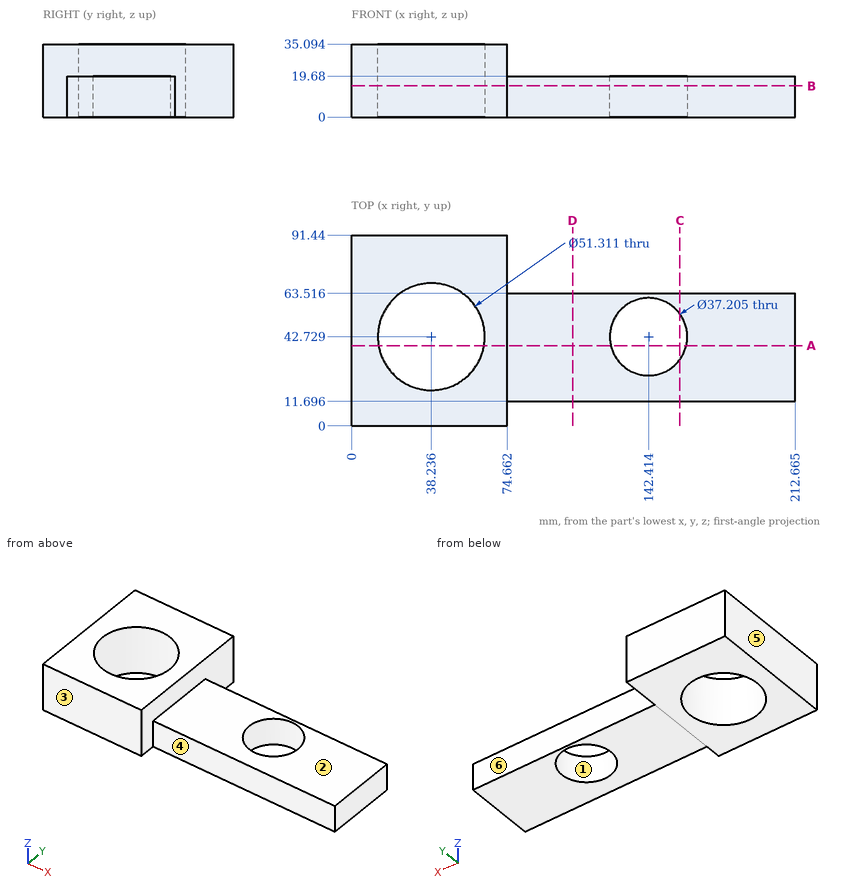
The figure shows three views and two pictorial views of one solid part (mm, origin at its lowest corner). Answer the questions. A direction names the side the tool comes from. Round coordinates to 2 decimals unless told otherwise and drop trailing zeros. Write each loop counter-clockwise with the first axis right and the second up, starting at its lowest first coordinate (ties: lowest second). Pieces come first, ordered by that corner, then holes. Notation, with made-up numbers: M 22,-20.75 L 77,-20.75 A32 cw 77,14.25 Z; hole C -15.5,-32 d10. An arc over 180 degrees is marked long. Use a Markdown table: item, result.
1) Which of the six approach directions +Z, -Z, +X, -X, +Y, -Y give full straight-line access (tool end or side, diameter ignored) to the marked faces 4, 5 and 6?
Taken from the geometry:
| item | result |
|---|---|
| face 4 | +Z, -Z, +X, -Y |
| face 5 | +Z, -Z, -X, +Y, -Y |
| face 6 | +Z, -Z, +X, +Y |
2) The part is cut by section D-D on x = 106. Give the vertices of the cut face in (y, z), plus the area to 3 significant figures.
Taken from the geometry:
| item | result |
|---|---|
| outline | M 11.7,0 L 63.52,0 L 63.52,19.68 L 11.7,19.68 Z |
| area | 1,020 mm2 |
3) The part is cut by section B-B on z = 15. Give the vertices of the cut face in (x, y) (1 decimal), plus the area to 3 significant figures.
Taken from the geometry:
| item | result |
|---|---|
| outline | M 0,0 L 74.7,0 L 74.7,11.7 L 212.7,11.7 L 212.7,63.5 L 74.7,63.5 L 74.7,91.4 L 0,91.4 Z; hole C 38.2,42.7 d51.3; hole C 142.4,42.7 d37.2 |
| area | 10,800 mm2 |
4) Determine the mould class of the marked faces 1, 2 and 3 for opening direction Y: pulls with the +Y half, pulls with the -Y half, needs draft (parallel to the pull), parting line crosses it, or undercut.
Taken from the geometry:
| item | result |
|---|---|
| face 1 | undercut |
| face 2 | needs draft |
| face 3 | pulls with the -Y half |
5) The part is cut by section A-A on y = 38.5. Give the vertices of the cut face in (x, z) (1 decimal).
Taken from the geometry:
| item | result |
|---|---|
| outline | M 0,0 L 12.9,0 L 12.9,35.1 L 0,35.1 Z; M 63.5,0 L 124.3,0 L 124.3,19.7 L 74.7,19.7 L 74.7,35.1 L 63.5,35.1 Z; M 160.5,0 L 212.7,0 L 212.7,19.7 L 160.5,19.7 Z |
6) Flat-ended cylindrical pins translate along their axes: pin 1 (8 mm diameter, centred on x = 81.5, y = 70.5, fed in from +Z); pin 2 (6 mm diameter, centred on x = 28.5, z = 16.5, fed in from -Y); pin 3 (8 mm diameter, centred on x = 170, y = 17, fed in from +Z); pin 4 (3 mm diameter, centred on y = 73.5, z = 14, fed in from +X). Find the tip coordinate at first contact, or state that the pin passes through.
Taken from the geometry:
| item | result |
|---|---|
| pin 1 | passes through |
| pin 2 | stops at y = 0 |
| pin 3 | stops at z = 19.68 |
| pin 4 | stops at x = 74.66 |
7) The part is cut by section C-C on x = 157.5. Give the vertices of the cut face in (y, z) (1 decimal).
Taken from the geometry:
| item | result |
|---|---|
| outline | M 11.7,0 L 31.8,0 L 31.8,19.7 L 11.7,19.7 Z; M 53.6,0 L 63.5,0 L 63.5,19.7 L 53.6,19.7 Z |
8) Consider line 1 (X direction, y = 40.5, z = 19) (1 decimal); line 2 (X direction, y = 15, z = 24); line 3 (Z direction, x = 182, y = 38). Determine where each line is inside the solid, lowest interval first. Write a range as [from, to].
Taken from the geometry:
| item | result |
|---|---|
| line 1 | x = [0, 12.7], [63.8, 123.9], [160.9, 212.7] |
| line 2 | x = [0, 74.66] |
| line 3 | z = [0, 19.68] |
